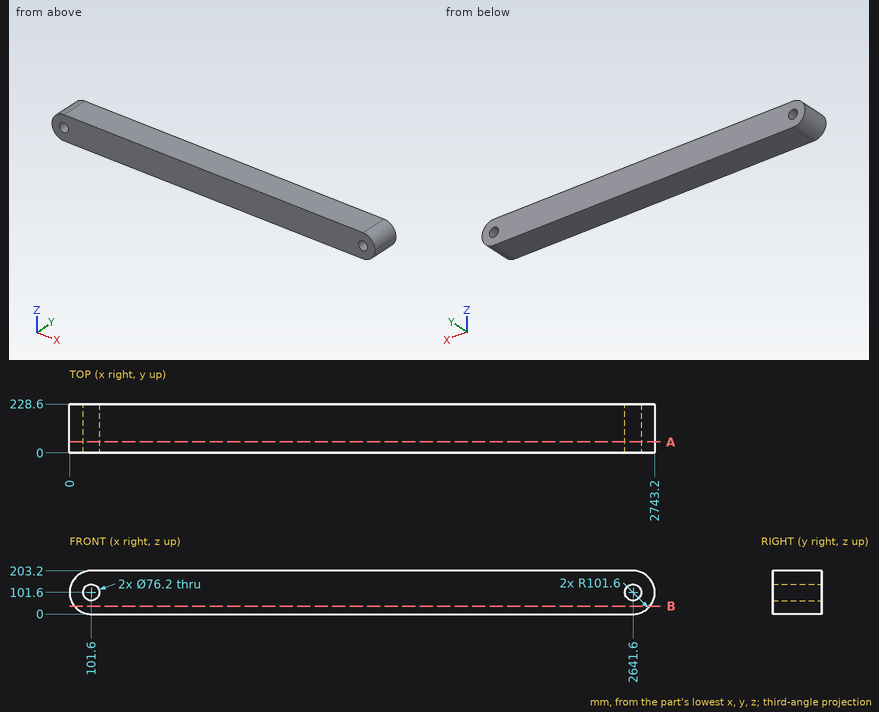
Could you check a few things on this drawing? It's one solid part, dimensions in mm from its lowest x, y, z. Round coordinates to 2 decimals unless told otherwise and drop trailing zeros. Loops run counter-clockwise (first coordinate to the right, second up) from the corner with the lowest first, then second, coordinate; pieces in that order, holes last. Notation, with made-up numbers: M 49,60.5 L 102,60.5 A28 cw 102,96.5 Z; hole C 78,57 d9. An arc over 180 degrees is marked long. Write each question's results on one line, items separated by ' | '. Start each with the question number.
(1) I want a section at B-B (z = 38). Please give me the cut outline in (x, y), then the cut area to 3 significant figures.
(2) Will these pins go through, and if not, where does the flat tip stop? P1, Ø1.5, axis at x = 1857.5, z = 24, coming from the -Y side; P2, Ø2, axis at y = 152, z = 173.5, coming from the +X side; P3, Ø5, axis at y = 159.5, z = 181.5, coming from the +X side; P4, Ø1.5, axis at y = 41, z = 87, coming from the -X side.
(3) If I drill on probe 1 along X at (y, z) = (158, 101); probe 2 along X at (y, z) = (219, 97); probe 3 along Z at (x, y) = (101.6, 57.5), over which ranges is the centre line in solid material (lowest first)? Write a range as from..to.
(4) I want a section at A-A (y = 51). Please give me the cut outline in (x, z).
Solved:
1) outline: M 22.37,0 L 2720.83,0 L 2720.83,228.6 L 22.37,228.6 Z | area: 617,000 mm²
2) P1: stops at y = 0 | P2: stops at x = 2714.37 | P3: stops at x = 2707.42 | P4: stops at x = 0.95
3) probe 1: x = 0..63.5, 139.7..2603.5, 2679.7..2743.2 | probe 2: x = 0.1..63.78, 139.42..2603.78, 2679.42..2743.1 | probe 3: z = 0..63.5, 139.7..203.2
4) outline: M 101.6,0 L 2641.6,0 A101.6 ccw 2641.6,203.2 L 101.6,203.2 A101.6 ccw Z; hole C 101.6,101.6 d76.2; hole C 2641.6,101.6 d76.2
